from build123d import *

# Parameters (mm, degrees)
BOSS_EXTRU_1_DEPTH                            = 70
TROU_POUR_TARAUDAGE_POUR_TROU_TARAUD_M1_D     = 10.2
D_GAGEMENT_M121_D                             = 13.5
D_GAGEMENT_M121_DEPTH                         = 40
D_GAGEMENT_M121_TIP                           = 4.055809178
CONG_2_R                                      = 20
ESQUISSE8_R                                   = 10
ENL_V_MAT_EXTRU_2_DEPTH                       = 89
ENL_V_MAT_EXTRU_3_DEPTH                       = 49
CONG_3_R                                      = 4
ESQUISSE10_R                                  = 20
ENL_V_MAT_EXTRU_4_DEPTH                       = 2
TROU_POUR_TARAUDAGE_POUR_TROU_TARAUD_M5_D     = 4.2
TROU_POUR_TARAUDAGE_POUR_TROU_TARAUD_M5_DEPTH = 8
TROU_POUR_TARAUDAGE_POUR_TROU_TARAUD_M5_TIP   = 1.2618073
ESQUISSE15_R                                  = 6
ENL_V_MAT_EXTRU_5_DEPTH                       = 15
CONG_4_R                                      = 3
ENL_V_MAT_EXTRU_6_DEPTH                       = 45
CONG_5_R                                      = 20
CONG_6_R                                      = 6
TROU_POUR_TARAUDAGE_POUR_TROU_TARAUD_2_D      = 4.2
TROU_POUR_TARAUDAGE_POUR_TROU_TARAUD_2_DEPTH  = 30
TROU_POUR_TARAUDAGE_POUR_TROU_TARAUD_2_TIP    = 1.2618073
TROU_POUR_TARAUDAGE_POUR_TROU_TARAUD_M4_D     = 3.3
TROU_POUR_TARAUDAGE_POUR_TROU_TARAUD_M4_DEPTH = 8
TROU_POUR_TARAUDAGE_POUR_TROU_TARAUD_M4_TIP   = 0.991420021
CHANFREIN2_SIZE                               = 0.5
CONG_7_R                                      = 6


with BuildPart() as part:
    # Esquisse1 → Boss.-Extru.1 (new body)
    with BuildSketch(Plane.XY):
        Polygon((32, 35), (-32, 35), (-50, 3.823085464), (-50, -74), (50, -74), (50, 3.823085464), align=None)
    extrude(amount=BOSS_EXTRU_1_DEPTH)

    # Trou pour taraudage pour trou taraudé M121 (through all)
    with Locations(Plane(origin=(0, -30, 0), x_dir=(-1, 0, 0), z_dir=(0, 0, -1))):
        with Locations((-27.189233611, 42.678547852), (0, 30)):
            Hole(TROU_POUR_TARAUDAGE_POUR_TROU_TARAUD_M1_D / 2)

    # Dégagement M121
    with Locations(Plane(origin=(0, 30, 0), x_dir=(1, 0, 0), z_dir=(0, 0, -1))):
        with Locations((27.189233611, 17.321452148)):
            Hole(D_GAGEMENT_M121_D / 2, depth=D_GAGEMENT_M121_DEPTH)
            with Locations((0, 0, -(D_GAGEMENT_M121_DEPTH + D_GAGEMENT_M121_TIP / 2))):  # 118° drill point
                Cone(0, D_GAGEMENT_M121_D / 2, D_GAGEMENT_M121_TIP, mode=Mode.SUBTRACT)

    # Congé2
    cong_2_edges = [part.edges().sort_by_distance(p)[0] for p in [
        (-50, 3.823085464, 35),
        (-32, 35, 35),
        (32, 35, 35),
        (50, 3.823085464, 35),
    ]]
    fillet(cong_2_edges, radius=CONG_2_R)

    # Esquisse8 → Enlèv. mat.-Extru.2 (cut)
    with BuildSketch(Plane.XZ.offset(74)):
        with Locations((-18, 29)):
            Circle(ESQUISSE8_R)
    extrude(amount=-ENL_V_MAT_EXTRU_2_DEPTH, mode=Mode.SUBTRACT)

    # Esquisse9 → Enlèv. mat.-Extru.3 (cut)
    with BuildSketch(Plane.XZ.offset(74)):
        Polygon((-46.500001617, 0.499996766), (-46.500001617, 57.5), (10.499998383, 57.5), (10.499998383, 0.500003234), (10.499998383, 0), (-46.500001617, 0), align=None)
        with BuildLine():
            Line((38, 56.7), (38, 45))
            Line((38, 45), (10, 45))
            Line((10, 45), (10, 56.7))
            ThreePointArc((10, 56.7), (12.928932188, 63.771067812), (20, 66.7))
            Line((20, 66.7), (28, 66.7))
            ThreePointArc((28, 66.7), (35.071067812, 63.771067812), (38, 56.7))
        make_face()
    extrude(amount=-ENL_V_MAT_EXTRU_3_DEPTH, mode=Mode.SUBTRACT)

    # Congé3
    cong_3_edges = [part.edges().sort_by_distance(p)[0] for p in [
        (-46.500001617, -49.5, 57.5),
    ]]
    fillet(cong_3_edges, radius=CONG_3_R)

    # Esquisse10 → Enlèv. mat.-Extru.4 (cut)
    with BuildSketch(Plane.XZ.offset(25)):
        with Locations((-18, 29)):
            Circle(ESQUISSE10_R)
    extrude(amount=-ENL_V_MAT_EXTRU_4_DEPTH, mode=Mode.SUBTRACT)

    # Trou pour taraudage pour trou taraud_ M5
    with Locations(Plane(origin=(0, -25, 0), x_dir=(-1, 0, 0), z_dir=(0, -1, 0))):
        with Locations((-5.57, -52.57), (41.57, -5.43), (41.57, -52.57), (-5.57, -5.43), (18, -29)):
            Hole(TROU_POUR_TARAUDAGE_POUR_TROU_TARAUD_M5_D / 2, depth=TROU_POUR_TARAUDAGE_POUR_TROU_TARAUD_M5_DEPTH)
            with Locations((0, 0, -(TROU_POUR_TARAUDAGE_POUR_TROU_TARAUD_M5_DEPTH + TROU_POUR_TARAUDAGE_POUR_TROU_TARAUD_M5_TIP / 2))):  # 118° drill point
                Cone(0, TROU_POUR_TARAUDAGE_POUR_TROU_TARAUD_M5_D / 2, TROU_POUR_TARAUDAGE_POUR_TROU_TARAUD_M5_TIP, mode=Mode.SUBTRACT)

    # Esquisse14 → Enlèvement de matière-Révolution2 (revolve, cut)
    with BuildSketch(Plane(origin=(0, 0, 0), x_dir=(0, 0, -1), z_dir=(1, 0, 0))):
        Polygon((0, 0), (-70, 0), (-70, 24.5), (-64, 24.5), (-64, 21), (-56, 21), (-56, 16), (-46, 16), (-46, 12.5), (-14.998685055, 12.5), (-14.998685055, 14), (0.001314945, 14), align=None)
    revolve(axis=Axis((0, 0, 0), (0, 0, 1)), mode=Mode.SUBTRACT)

    # Esquisse15 → Enlèv. mat.-Extru.5 (cut)
    with BuildSketch(Plane.XY.offset(70)):
        with Locations((27.189233611, 12.678547852)):
            Circle(ESQUISSE15_R)
    extrude(amount=-ENL_V_MAT_EXTRU_5_DEPTH, mode=Mode.SUBTRACT)

    # Congé4
    cong_4_edges = [part.edges().sort_by_distance(p)[0] for p in [
        (23.032598632, 8.351610639, 67),
        (21.20277394, 12.275682353, 67),
    ]]
    fillet(cong_4_edges, radius=CONG_4_R)

    # Esquisse16 → Enlèv. mat.-Extru.6 (cut)
    with BuildSketch(Plane(origin=(0, 0, 0), x_dir=(-1, 0, 0), z_dir=(0, 0, -1))):
        with BuildLine():
            Line((-38, -74), (-20.439233611, -74))
            Line((-20.439233611, -74), (-10.499998383, -74))
            Line((-10.499998383, -74), (-10.499998383, -25))
            Line((-10.499998383, -25), (-19.189233611, -25))
            Line((-19.189233611, -25), (-19.189233611, 12.678547852))
            ThreePointArc((-19.189233611, 12.678547852), (-25.11868125, 20.405954463), (-34.117436841, 16.678547852))
            Line((-34.117436841, 16.678547852), (-38, 9.953751198))
            Line((-38, 9.953751198), (-38, -74))
        make_face()
    extrude(amount=-ENL_V_MAT_EXTRU_6_DEPTH, mode=Mode.SUBTRACT)

    # Congé5
    cong_5_edges = [part.edges().sort_by_distance(p)[0] for p in [
        (38, 9.953751198, 22.5),
    ]]
    fillet(cong_5_edges, radius=CONG_5_R)

    # Congé6
    cong_6_edges = [part.edges().sort_by_distance(p)[0] for p in [
        (19.189233611, -25, 22.5),
    ]]
    fillet(cong_6_edges, radius=CONG_6_R)

    # Trou pour taraudage pour trou taraud 2
    with Locations(Plane(origin=(0, -74, 0), x_dir=(-1, 0, 0), z_dir=(0, -1, 0))):
        with Locations((44, -64), (-44, -64), (-44, -15)):
            Hole(TROU_POUR_TARAUDAGE_POUR_TROU_TARAUD_2_D / 2, depth=TROU_POUR_TARAUDAGE_POUR_TROU_TARAUD_2_DEPTH)
            with Locations((0, 0, -(TROU_POUR_TARAUDAGE_POUR_TROU_TARAUD_2_DEPTH + TROU_POUR_TARAUDAGE_POUR_TROU_TARAUD_2_TIP / 2))):  # 118° drill point
                Cone(0, TROU_POUR_TARAUDAGE_POUR_TROU_TARAUD_2_D / 2, TROU_POUR_TARAUDAGE_POUR_TROU_TARAUD_2_TIP, mode=Mode.SUBTRACT)

    # Trou pour taraudage pour trou taraudé M41
    with Locations(Plane(origin=(0, 0, 0), x_dir=(-1, 0, 0), z_dir=(0, 0, -1))):
        with Locations((44, -14), (30.845299462, 25), (-30.845299462, 25), (-44, -68)):
            Hole(TROU_POUR_TARAUDAGE_POUR_TROU_TARAUD_M4_D / 2, depth=TROU_POUR_TARAUDAGE_POUR_TROU_TARAUD_M4_DEPTH)
            with Locations((0, 0, -(TROU_POUR_TARAUDAGE_POUR_TROU_TARAUD_M4_DEPTH + TROU_POUR_TARAUDAGE_POUR_TROU_TARAUD_M4_TIP / 2))):  # 118° drill point
                Cone(0, TROU_POUR_TARAUDAGE_POUR_TROU_TARAUD_M4_D / 2, TROU_POUR_TARAUDAGE_POUR_TROU_TARAUD_M4_TIP, mode=Mode.SUBTRACT)

    # Chanfrein2
    chanfrein2_edges = [part.edges().sort_by_distance(p)[0] for p in [
        (50, -37.767949192, 70),
        (0, -14, 0),
        (0, -12.5, 46),
        (0, -21, 64),
        (0, -16, 56),
        (0, -12.5, 14.998685055),
        (-22.204540782, -10.354147413, 70),
        (29.261261506, 18.309418158, 70),
        (20.385817669, 15.512623626, 70),
        (24.987110138, 5.645120084, 70),
        (-50, -37.767949192, 70),
        (-42.547005384, 16.732050808, 70),
        (42.547005384, 16.732050808, 70),
        (0, 35, 70),
        (30.452994616, 32.320508076, 70),
        (-30.452994616, 32.320508076, 70),
        (49.318516526, 3.640482517, 70),
        (-49.318516526, 3.640482517, 70),
    ]]
    chamfer(chanfrein2_edges, length=CHANFREIN2_SIZE)

    # Congé7
    cong_7_edges = [part.edges().sort_by_distance(p)[0] for p in [
        (10.032051364, -49.5, 57.5),
    ]]
    fillet(cong_7_edges, radius=CONG_7_R)


solid = part.part
Here's how the part is built. I have some questions about the finished solid (model axes, mm). A direction names the side the tool comes from. Round coordinates to 2 decimals unless told otherwise and drop trailing zeros.
1. For faces 5 (the cylindrical face through (32.912, 14.481, 62.352)), 6 (the flat face through (-19, -50, 57.5)), 7 (the cylindrical face through (5.11, -20.94, 54.62)), which set-ups out of +Z, -Z, +X, -X, +Y, -Y let a thin tool reach every point of the face, with its end or its side?
2. If we mould it in two halves opening along Y, with no side actions, what happens to faces 1 (the cylindrical face through (43.727, -58.79, 12.918)), 2 (the flat face through (11, -13, 56)), 3 (the flat face through (-13.1, -1.3, 46)), 4 (the cylindrical face through (17.385, -23.289, 22.815))? For each: released by +Y, released by -Y, zero draft, split by the parting line, or undercut.
3. I need wall thicknesses on L1, parallel to X at y = -21.5, z = 52.57; L2, parallel to Y at x = 0, z = 7; L3, parallel to Z at x = 5.57, y = -18.25. Which ranges of each line are inside material? Lowest first, please.
4. Will these pins go through, and if not, where does the flat tip stop? pin 1 Ø1 at (x, y) = (8.5, -27.5) entering from -Z; pin 2 Ø2.5 at (x, z) = (-41.57, 5.43) entering from +Y; pin 3 Ø2.5 at (x, y) = (-44, -14) entering from -Z.
Answer sheet:
1. face 5: +Z
1. face 6: -Z, -Y
1. face 7: -Y
2. face 1: zero draft
2. face 2: undercut
2. face 3: undercut
2. face 4: released by -Y
3. L1: x = -50 to -43.67, -39.47 to 3.47, 7.67 to 50
3. L2: y = -25 to -14, 14 to 35
3. L3: z = 0 to 3.33, 7.53 to 50.47, 54.67 to 56
4. pin 1: stops at z = 58.04
4. pin 2: stops at y = 20.59
4. pin 3: stops at z = 8.24
